For this review, take the finished solid that the model builds, in its own axes (mm). A direction names the side the tool comes from. Give positions to 0.01 mm unless a question says otherwise; leave off trailing zeros. Order: outer loops, then holes, each group sorted by start corner. A loop starts at its lowest first (then second) coordinate and runs counter-clockwise, first axis right, second up. Notation, with made-up numbers: (-4, -7.5) - (47, -7.5) arc R27 cw to (47, 12.5) - close; hole circle Ø5 at (72, 10). An arc over 180 degrees is marked (long way). Use a Markdown table: item, result. Add a question column.
1) We need section C-C on x = 42. Write out the cut boundary in (y, z), then the cut area to 3 significant figures.
2) Wall thickness on L1, parallel to X at y = -23, z = 0; L2, parallel to Z at x = 155, y = 25; L3, parallel to Z at x = 155, y = -24.25: over which ranges is each line inside the solid? List them lowest first.
3) Clearance check with flat-ended pins moving along their axes: P1, Ø24, axis at x = 155, z = 0, coming from the +Y side; P2, Ø6, axis at x = 62, y = 22, coming from the +Z side; P3, Ø12, axis at y = -22, z = 18, coming from the -X side; P4, Ø1.5, axis at x = 100.5, z = 3.5, coming from the +Y side. State where each tip first meets the part, or that it passes through.
4) We need section B-B on x = 155. Write out the cut boundary in (y, z), then the cut area to 3 significant figures.
5) We need section A-A on z = 0. Write out the cut boundary in (x, y), then the cut area to 3 significant figures.
6) Mouldability with a two-part tool opening along Y and no side actions: class faces 4 (the face through (64, 0, 25)), 5 (the face through (125, 0, 0)), 6 (the face through (81, -30, 0)) as released by +Y, released by -Y, zero draft, split by the parting line, or undercut.
7) Machinability: for faces 1 (the face through (0, -6, -5)), 2 (the face through (81, 30, 0)), 3 (the face through (147, -16.583, 0)), which of the approach directions +Z, -Z, +X, -X, +Y, -Y give a long, thin tool a straight path to every point of the face, cutting with its end or side? Answer none if there is none.
8) We need section D-D on y = -14. Write out the cut boundary in (x, z).
```python
from build123d import *

# Parameters (mm, degrees)
BOSS_EXTRUDE1_DEPTH = 170
SKETCH5_R           = 7.5
BOSS_EXTRUDE2_DEPTH = 20
CUT_EXTRUDE1_DEPTH  = 180.722007556
SKETCH8_R           = 7.5
CUT_EXTRUDE2_DEPTH  = 48.5
FILLET1_R           = 6


with BuildPart() as part:
    # Sketch1 → Boss-Extrude1 (new body)
    with BuildSketch(Plane(origin=(0, 0, 0), x_dir=(0, 0, -1), z_dir=(1, 0, 0))):
        with BuildLine():
            Line((-25, 16.583123952), (-25, -16.583123952))
            ThreePointArc((-25, -16.583123952), (0, -30), (25, -16.583123952))
            Line((25, -16.583123952), (25, 16.583123952))
            ThreePointArc((25, 16.583123952), (0, 30), (-25, 16.583123952))
        make_face()
    extrude(amount=BOSS_EXTRUDE1_DEPTH)

    # Sketch5 → Boss-Extrude2 (add)
    with BuildSketch(Plane.ZY):
        with Locations(Location((0, 0, 0), (0, 0, 180))):
            Circle(SKETCH5_R)
    extrude(amount=BOSS_EXTRUDE2_DEPTH)

    # Sketch7 → Cut-Extrude1 (cut, through all)
    with BuildSketch(Plane(origin=(0, 0, -25), x_dir=(-1, 0, 0), z_dir=(0, 0, -1))):
        with BuildLine():
            Line((-180, -16.583123952), (-130, -16.583123952))
            ThreePointArc((-130, -16.583123952), (-125, 0), (-130, 16.583123952))
            Line((-130, 16.583123952), (-180, 16.583123952))
            ThreePointArc((-180, 16.583123952), (-185, 0), (-180, -16.583123952))
        make_face()
    extrude(amount=-CUT_EXTRUDE1_DEPTH, mode=Mode.SUBTRACT)

    # Sketch8 → Cut-Extrude2 (cut, symmetric)
    with BuildSketch(Plane(origin=(0, 0, 0), x_dir=(1, 0, 0), z_dir=(0, 1, 0))):
        with Locations(Location((155, 0, 0), (0, 0, 270))):
            Circle(SKETCH8_R)
    extrude(amount=CUT_EXTRUDE2_DEPTH, both=True, mode=Mode.SUBTRACT)

    # Fillet1
    fillet1_edges = [part.edges().sort_by_distance(p)[0] for p in [
        (170, 30, 0),
        (170, 16.583123952, 0),
        (170, -16.583123952, 0),
        (170, -30, 0),
    ]]
    fillet(fillet1_edges, radius=FILLET1_R)


solid = part.part
```
Checked values:
| question | item | result |
|---|---|---|
| 1 | outline | (-16.58, -25) - (16.58, -25) arc R30 ccw to (16.58, 25) - (-16.58, 25) arc R30 ccw to start |
| 1 | area | 2,600 mm² |
| 2 | L1 | 0 to 147.5, 162.5 to 170 |
| 2 | L2 | -16.58 to -7.5, 7.5 to 16.58 |
| 2 | L3 | -17.66 to -7.5, 7.5 to 17.66 |
| 3 | P1 | y = 30 |
| 3 | P2 | z = 23.22 |
| 3 | P3 | x = 0 |
| 3 | P4 | y = 29.87 |
| 4 | outline | (-29.05, -7.5) arc R30 ccw to (-16.58, -25) - (-16.58, -7.5) - close; (-29.05, 7.5) - (-16.58, 7.5) - (-16.58, 25) arc R30 ccw to start; (16.58, -25) arc R30 ccw to (29.05, -7.5) - (16.58, -7.5) - close; (16.58, 7.5) - (29.05, 7.5) arc R30 ccw to (16.58, 25) - close |
| 4 | area | 551 mm² |
| 5 | outline | (-20, -7.5) - (0, -7.5) - (0, -30) - (147.5, -30) - (147.5, -16.58) - (130, -16.58) arc R30 cw to (130, 16.58) - (147.5, 16.58) - (147.5, 30) - (0, 30) - (0, 7.5) - (-20, 7.5) - close; (162.5, -30) - (164, -30) arc R6 ccw to (170, -24) - (170, -22.58) arc R6 ccw to (164, -16.58) - (162.5, -16.58) - close; (162.5, 16.58) - (164, 16.58) arc R6 ccw to (170, 22.58) - (170, 24) arc R6 ccw to (164, 30) - (162.5, 30) - close |
| 5 | area | 8,630 mm² |
| 6 | face 4 | zero draft |
| 6 | face 5 | undercut |
| 6 | face 6 | released by -Y |
| 7 | face 1 | -X |
| 7 | face 2 | +X, -X, +Y |
| 7 | face 3 | +Z, -Z, +X |
| 8 | outline | (0, -25) - (128.47, -25) - (128.47, 25) - (0, 25) - close |
